Geometry check sheet. Reference: drawing and pictorial views, mm from the part's lowest x, y, z. A direction names the side the tool comes from. Round coordinates to 2 decimals unless told otherwise and drop trailing zeros. Order: outer loops, then holes, each group sorted by start corner. A loop starts at its lowest first (then second) coordinate and runs counter-clockwise, first axis right, second up.
(1) Sectioned sample at C-C (x = 56.5). Record the boundary of the cut face in (y, z), plus the area to 3 significant figures.
(2) Material ranges on line 1 along X through (y, z) = (10.5, 5); line 2 along X through (y, z) = (21.5, 9.5); line 3 along Y through (x, z) = (19.5, 7.5) (3 decimals), recorded low to high.
(3) Sectioned sample at B-B (z = 14.25). Record the boundary of the cut face in (x, y) (3 decimals).
(4) Sectioned sample at A-A (y = 22.25). Record the boundary of the cut face in (x, z).
(5) Set-up check for the marked faces 5, 6 and 7: record each of +Z, -Z, +X, -X, +Y, -Y from which the full face is reachable in a straight line by a thin tool's end or side.
(6) Go/stop test with flat-tipped pins: pin 1 (8 mm diameter, centred on y = 20, z = 3.5, fed in from +X); pin 2 (10 mm diameter, centred on x = 18, z = 17.5, fed in from +Y) (3 decimals); pin 3 (5.5 mm diameter, centred on x = 50.5, z = 13.5, fed in from +Y). Record where each tip stops, or that it passes through.
(7) Sectioned sample at D-D (x = 24.5). Record the boundary of the cut face in (y, z) (3 decimals).
(8) Release check for a two-part mould opening along X. For the marked faces 1, 2, 3 and 4 record: +X half, -X half, draft (parallel to the pull), parting line (faces both ways), or undercut.
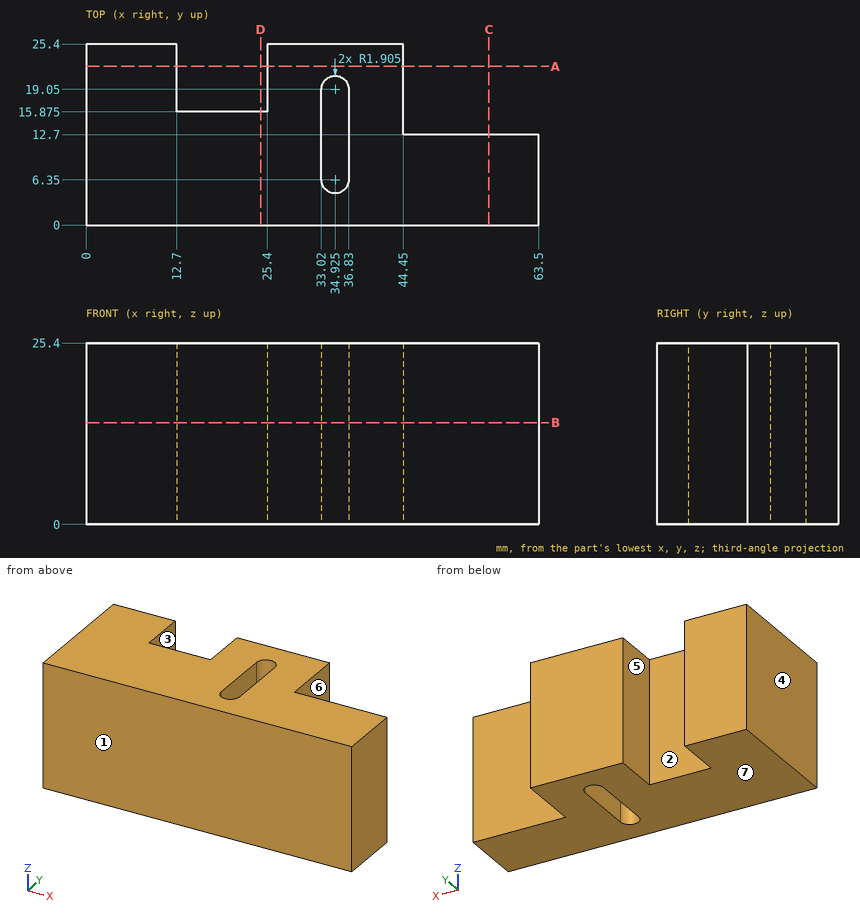
Answer below:
1. outline: (0, 0) - (12.7, 0) - (12.7, 25.4) - (0, 25.4) - close
1. area: 323 mm2
2. line 1: x = 0 to 33.02, 36.83 to 63.5
2. line 2: x = 0 to 12.7, 25.4 to 44.45
2. line 3: y = 0 to 15.875
3. outline: (0, 0) - (63.5, 0) - (63.5, 12.7) - (44.45, 12.7) - (44.45, 25.4) - (25.4, 25.4) - (25.4, 15.875) - (12.7, 15.875) - (12.7, 25.4) - (0, 25.4) - close; hole (33.02, 6.35) arc R1.905 ccw to (36.83, 6.35) - (36.83, 19.05) arc R1.905 ccw to (33.02, 19.05) - close
4. outline: (0, 0) - (12.7, 0) - (12.7, 25.4) - (0, 25.4) - close; (25.4, 0) - (44.45, 0) - (44.45, 25.4) - (25.4, 25.4) - close
5. face 5: +Z, -Z, +Y
5. face 6: +Z, -Z, +X, +Y
5. face 7: -Z, +X, -X, +Y, -Y
6. pin 1: stops at x = 44.45
6. pin 2: stops at y = 15.875
6. pin 3: stops at y = 12.7
7. outline: (0, 0) - (15.875, 0) - (15.875, 25.4) - (0, 25.4) - close
8. face 1: draft
8. face 2: undercut
8. face 3: undercut
8. face 4: -X half
